Part print with two shaded views. Sizes in mm from the minimum x, y, z corner. A direction names the side the tool comes from. Give positions to 0.01 mm unless a question says otherwise; leave off trailing zeros. Order: outer loops, then holes, each group sorted by start corner. A loop starts at its lowest first (then second) coordinate and runs counter-clockwise, first axis right, second up. Notation, with made-up numbers: M 37.25,-40 L 46.25,-40 A20 ccw 46.25,-2 Z; hole C 22.25,85.25 d5. An arc over 180 degrees is marked long. Return JSON: item names as keys, results as strings. Group by question number.
1. Slice it at A-A on y = 23.25. List the corners of the cut face in (x, z).
2. Slice it at B-B on x = 28. List the corners of the cut face in (y, z).
3. Pin check, flat tips, straight feed: pin 1 (4 mm diameter, centred on y = 15.5, z = 17.5, fed in from +X) (1 decimal); pin 2 (10 mm diameter, centred on x = 30, y = 11.5, fed in from +Z); pin 3 (6 mm diameter, centred on y = 18.5, z = 18, fed in from +X). Stop position of each tip, or through.
4. Slice it at C-C on z = 24.5. List the corners of the cut face in (x, y), then the cut area to 3 significant figures.
5. Wall check: probe 1 along Z at (x, y) = (26.5, 14); probe 2 along X at (y, z) = (3.5, 30.5); probe 3 along X at (y, z) = (19.75, 29). Give the ranges that are in metal, low to high. Write a range as [from, to].
6. 3-axis set-ups, long thin cutter, end or side, ignore diameter. For the marked faces 1 and 2: which of +Z, -Z, +X, -X, +Y, -Y reach the whole face in a straight line?
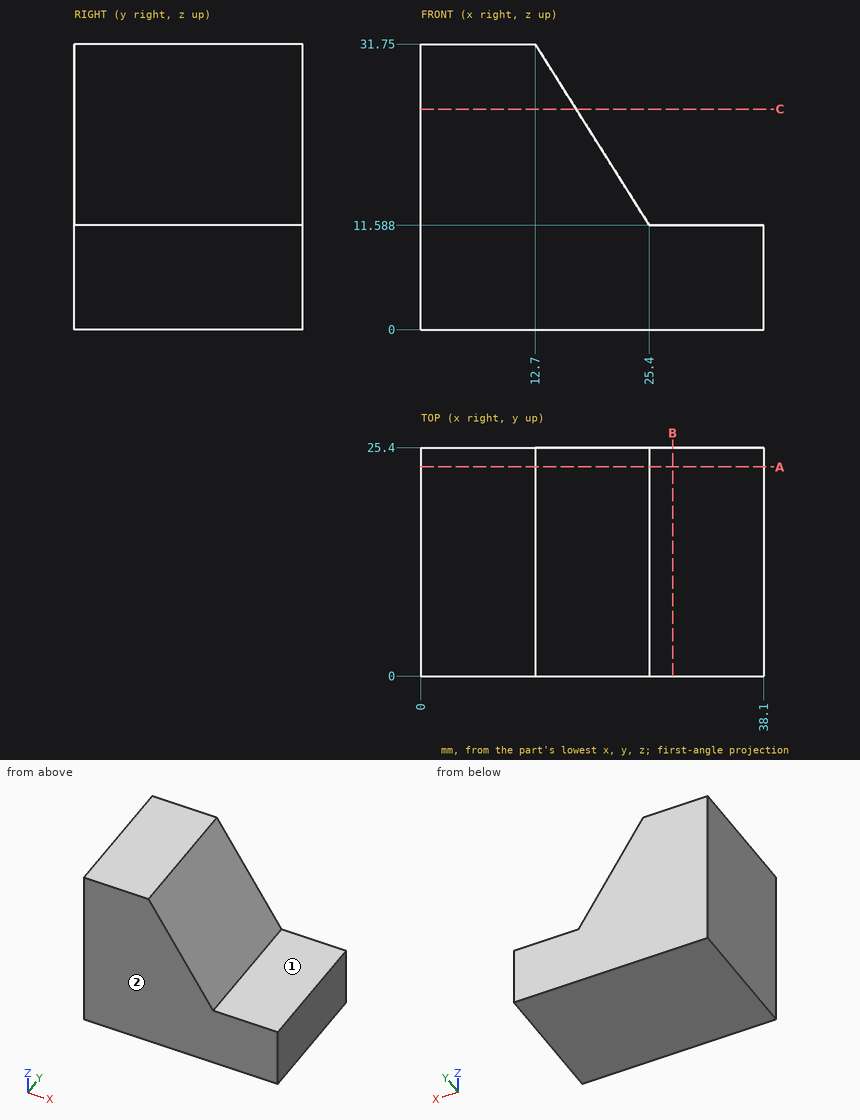
Result:
{
 "1": {"outline": "M 0,0 L 38.1,0 L 38.1,11.59 L 25.4,11.59 L 12.7,31.75 L 0,31.75 Z"},
 "2": {"outline": "M 0,0 L 25.4,0 L 25.4,11.59 L 0,11.59 Z"},
 "3": {"pin 1": "stops at x = 22.9", "pin 2": "stops at z = 12.22", "pin 3": "stops at x = 23.25"},
 "4": {"outline": "M 0,0 L 17.27,0 L 17.27,25.4 L 0,25.4 Z", "area": "439 mm2"},
 "5": {"probe 1": "z = [0, 11.59]", "probe 2": "x = [0, 13.49]", "probe 3": "x = [0, 14.43]"},
 "6": {"face 1": "+Z, +X, +Y, -Y", "face 2": "+Z, -Z, +X, -X, -Y"}
}
